CAD build for the part. Positions are in the model's coordinates, mm. Face numbers are marked on the shaded views. A direction names the side the tool comes from. Give positions to 0.01 mm unless a question says otherwise; leave off trailing zeros. Order: outer loops, then holes, each group sorted by start corner. A loop starts at its lowest first (then second) coordinate and runs counter-clockwise, first axis right, second up.
Item 1: Which spindle directions (+Z, -Z, +X, -X, +Y, -Y) get a long thin tool onto all of the face, cutting with end or side? Do the marked faces 4 and 5. Say none if no direction does.
Item 2: Band-saw the part on A-A on z = 0. Give the cut face in (x, y).
Item 3: Two-plate mould, pull along X, no slides. Class the marked faces 1, 2 and 3: released by +X, released by -X, zero draft, split by the parting line, or undercut.
Item 4: Wall check: L1, parallel to X at y = 2.75, z = 0; L2, parallel to Y at x = -14, z = 21.5; L3, parallel to X at y = 10.5, z = -28. Give the ranges that are in metal, low to high.
Item 5: Band-saw the part on D-D on y = 2. Give the cut face in (x, z), plus the area to 3 significant figures.
Item 6: Flat gauge pins, fed straight in: P1, Ø1.5, axis at x = -2.5, y = 2, coming from the -Z side; P2, Ø6, axis at y = 7.75, z = -29.71, coming from the +X side; P3, Ø2, axis at x = -20.5, y = 6.5, coming from the +Z side. Where does each tip first touch, or does it go through?
Item 7: Band-saw the part on C-C on y = 7.75. Give the cut face in (x, z).
Item 8: Band-saw the part on B-B on x = 0. Give the cut face in (y, z), plus the area to 3 significant figures.
```python
from build123d import *

# Parameters (mm, degrees)
BOSS_EXTRUDE1_DEPTH = 4
SKETCH2_W           = 3
SKETCH2_H           = 8
BOSS_EXTRUDE2_DEPTH = 7
SKETCH3_R           = 1.8
CUT_EXTRUDE1_DEPTH  = 62.847529316
FILLET1_R           = 4
FILLET2_R           = 10
FILLET3_R           = 1
FILLET4_R           = 1
SKETCH4_R           = 21.5
CUT_EXTRUDE2_DEPTH  = 46.764253326


with BuildPart() as part:
    # Sketch1 → Boss-Extrude1 (new body)
    with BuildSketch(Plane(origin=(0, 0, 0), x_dir=(1, 0, 0), z_dir=(0, 1, 0))):
        with BuildLine():
            Line((18.5, 33.213203436), (18.5, 22.978250586))
            ThreePointArc((18.5, 22.978250586), (0, 29.5), (-18.5, 22.978250586))
            Line((-18.5, 22.978250586), (-18.5, 33.213203436))
            Line((-18.5, 33.213203436), (-21.5, 33.213203436))
            Line((-21.5, 33.213203436), (-21.5, 20.199009877))
            ThreePointArc((-21.5, 20.199009877), (0, -29.5), (21.5, 20.199009877))
            Line((21.5, 20.199009877), (21.5, 33.213203436))
            Line((21.5, 33.213203436), (18.5, 33.213203436))
        make_face()
    extrude(amount=BOSS_EXTRUDE1_DEPTH)

    # Sketch2 → Boss-Extrude2 (add)
    with BuildSketch(Plane(origin=(0, 4, 0), x_dir=(1, 0, 0), z_dir=(0, 1, 0))):
        with Locations((-20, 29.213203436)):
            Rectangle(SKETCH2_W, SKETCH2_H)
        with Locations((20, 29.213203436)):
            Rectangle(SKETCH2_W, SKETCH2_H)
    extrude(amount=BOSS_EXTRUDE2_DEPTH)

    # Sketch3 → Cut-Extrude1 (cut, through all)
    with BuildSketch(Plane.ZY.offset(21.5)):
        with Locations(Location((-29.713203436, 7.75, 0), (0, 0, 180))):
            Circle(SKETCH3_R)
    extrude(amount=-CUT_EXTRUDE1_DEPTH, mode=Mode.SUBTRACT)

    # Fillet1
    fillet1_edges = [part.edges().sort_by_distance(p)[0] for p in [
        (-20, 11, -25.213203436),
        (-20, 11, -33.213203436),
        (20, 11, -25.213203436),
        (20, 11, -33.213203436),
        (20, 0, -33.213203436),
        (-20, 0, -33.213203436),
    ]]
    fillet(fillet1_edges, radius=FILLET1_R - 0.0001)  # a hair under: the kernel refuses the full size

    # Fillet2
    fillet2_edges = [part.edges().sort_by_distance(p)[0] for p in [
        (21.5, 2, -20.199009877),
        (-21.5, 2, -20.199009877),
    ]]
    fillet(fillet2_edges, radius=FILLET2_R)

    # Fillet3
    fillet3_edges = [part.edges().sort_by_distance(p)[0] for p in [
        (18.5, 2, -22.978250586),
        (-18.5, 2, -22.978250586),
    ]]
    fillet(fillet3_edges, radius=FILLET3_R)

    # Fillet4
    fillet4_edges = [part.edges().sort_by_distance(p)[0] for p in [
        (-20, 4, -25.213203436),
        (20, 4, -25.213203436),
    ]]
    fillet(fillet4_edges, radius=FILLET4_R)

    # Sketch4 → Cut-Extrude2 (cut, through all)
    with BuildSketch(Plane.XZ):
        with Locations(Location((0, 0, 0), (0, 0, 270))):
            Circle(SKETCH4_R)
    extrude(amount=-CUT_EXTRUDE2_DEPTH, mode=Mode.SUBTRACT)


solid = part.part
```
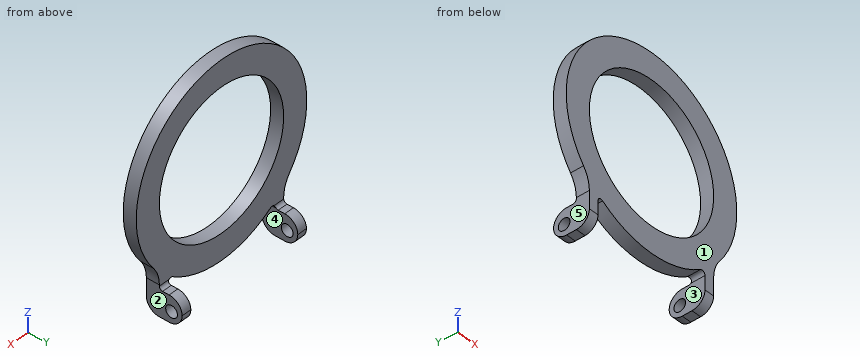
The answers:
1. face 4: -Z, +Y, -Y
1. face 5: -Z, -X, +Y, -Y
2. outline: (-29.5, 0) - (-21.5, 0) - (-21.5, 4) - (-29.5, 4) - close; (21.5, 0) - (29.5, 0) - (29.5, 4) - (21.5, 4) - close
3. face 1: zero draft
3. face 2: released by +X
3. face 3: undercut
4. L1: x = -29.5 to -21.5, 21.5 to 29.5
4. L2: y = 0 to 4
4. L3: x = -21.5 to -18.5, 18.5 to 21.5
5. outline: (-23.53, -17.8) arc R10 cw to (-21.5, -23.83) - (-21.5, -32.68) - (-18.5, -32.68) - (-18.5, -24.98) arc R1 cw to (-16.93, -24.16) arc R29.5 ccw to (16.93, -24.16) arc R1 cw to (18.5, -24.98) - (18.5, -32.68) - (21.5, -32.68) - (21.5, -23.83) arc R10 cw to (23.53, -17.8) arc R29.5 ccw (long way) to start; hole circle Ø43 at (0, 0)
5. area: 1,350 mm2
6. P1: stops at z = -29.45
6. P2: stops at x = 21.5
6. P3: stops at z = -25.21
7. outline: (-21.5, -33.14) - (-18.5, -33.14) - (-18.5, -31.51) - (-21.5, -31.51) - close; (-21.5, -27.91) - (-18.5, -27.91) - (-18.5, -25.28) - (-21.5, -25.28) - close; (18.5, -33.14) - (21.5, -33.14) - (21.5, -31.51) - (18.5, -31.51) - close; (18.5, -27.91) - (21.5, -27.91) - (21.5, -25.28) - (18.5, -25.28) - close
8. outline: (0, -29.5) - (4, -29.5) - (4, -21.5) - (0, -21.5) - close; (0, 21.5) - (4, 21.5) - (4, 29.5) - (0, 29.5) - close
8. area: 64.0 mm2
